from build123d import *

# Parameters (mm, degrees)
SKETCH3_R           = 2
SKETCH3_R_2         = 1.5
SKETCH4_R           = 2
SKETCH4_R_2         = 1.5
BOSS_EXTRUDE1_DEPTH = 20


with BuildPart() as part:
    # Sweep1: sweep along a path in Sketch2
    with BuildLine(Plane(origin=(0, 0, 0), x_dir=(1, 0, 0), z_dir=(0, 1, 0))) as sweep1_path:
        Line((-41, 0), (-41, -20))
        ThreePointArc((-41, -20), (-38.071067812, -27.071067812), (-31, -30))
        Line((-31, -30), (31, -30))
        ThreePointArc((31, -30), (38.071067812, -27.071067812), (41, -20))
        Line((41, -20), (41, 0))
    # Sketch3 → Sweep1 (sweep)
    with BuildSketch(Plane.XY):
        with Locations((-41, 0)):
            Circle(SKETCH3_R)
        with Locations((-41, 0)):
            Circle(SKETCH3_R_2, mode=Mode.SUBTRACT)
    sweep(path=sweep1_path.line)

    # Sketch4 → Boss-Extrude1 (add)
    with BuildSketch(Plane(origin=(0, 0, 0), x_dir=(1, 0, 0), z_dir=(0, 1, 0))):
        with Locations(Location((0, -30, 0), (0, 0, 270))):
            Circle(SKETCH4_R)
        with Locations(Location((0, -30, 0), (0, 0, 90))):
            Circle(SKETCH4_R_2, mode=Mode.SUBTRACT)
    extrude(amount=BOSS_EXTRUDE1_DEPTH)


solid = part.part
Check sheet for the modelled part. Datum: model origin and axes. Units: mm. A direction names the side the tool comes from. Give positions to 0.01 mm unless a question says otherwise; leave off trailing zeros. Loops run counter-clockwise (first coordinate to the right, second up) from the corner with the lowest first, then second, coordinate; pieces in that order, holes last. Notation, with made-up numbers: M 55,2 L 91,2 A24 cw 91,12 Z; hole C -4,41 d8. An arc over 180 degrees is marked long. Return JSON: item names as keys, results as strings. Group by question number.
1. Tool access check on faces 5 (the flat face through (1.7, 0, 29.9)), 6 (the cylindrical face through (43, 0, 10)). Record the directions out of +Z, -Z, +X, -X, +Y, -Y that give a thin tool (end or side, any length) a straight path to the whole face; none if there is none.
2. Thickness scan on L1, parallel to Z at x = 2.5, y = 0; L2, parallel to Y at x = 41, z = 12.5; L3, parallel to X at y = 0.5, z = 14. Record the ranges inside material, lowest first.
3. Go/stop test with flat-tipped pins: pin 1 (3 mm diameter, centred on y = 2, z = 6, fed in from -X); pin 2 (12 mm diameter, centred on x = -7.5, z = 21.5, fed in from +Y); pin 3 (0.6 mm diameter, centred on x = 0.5, z = 30.5, fed in from -Y); pin 4 (2 mm diameter, centred on y = 2.5, z = 25, fed in from +X). Record where each tip stops, or that it passes through.
4. Cross-section at A-A on z = 14. Record the boundary of the cut face in (x, y).
5. Cross-section at B-B on x = -24.5. Record the boundary of the cut face in (y, z).
6. Cross-section at D-D on z = 27. State how many separate pieces and enclosed holes the cut face has, plus the area to 3 significant figures.
7. Mould release check, pull along Y, two halves, no side actions. Record for faces 1 (the cylindrical face through (42.5, 0.07, 9.86)), 2 (the cylindrical face through (-43, 0, 10)), 3 (the cylindrical face through (-2, 1, 30)), 4 (the cylindrical face through (-0.766, 9.86, 31.847)): released by +Y, released by -Y, zero draft, split by the parting line, or undercut.
Return value:
{
 "1": {"face 5": "none", "face 6": "-Z"},
 "2": {"L1": "28 to 28.5, 31.5 to 32", "L2": "-2 to -1.5, 1.5 to 2", "L3": "-42.94 to -42.41, -39.59 to -39.06, 39.06 to 39.59, 42.41 to 42.94"},
 "3": {"pin 1": "x = -42.94", "pin 2": "through", "pin 3": "y = -1.99", "pin 4": "x = 41.24"},
 "4": {"outline": "C -41,0 d4; C 41,0 d4; hole C -41,0 d3; hole C 41,0 d3"},
 "5": {"outline": "C 0,30 d4; hole C 0,30 d3"},
 "6": {"separate pieces": "2", "enclosed holes": "2", "area": "16.3 mm^2"},
 "7": {"face 1": "undercut", "face 2": "split by the parting line", "face 3": "undercut", "face 4": "zero draft"}
}
